Read the model definition and answer for the solid it produces. Units are mm, in the model's axes. A direction names the side the tool comes from. Round coordinates to 2 decimals unless told otherwise and drop trailing zeros. Loops run counter-clockwise (first coordinate to the right, second up) from the corner with the lowest first, then second, coordinate; pieces in that order, holes last. Notation, with made-up numbers: M 54.5,-10 L 63.5,-10 A32 cw 63.5,25 Z; hole C 73.25,41.25 d11. An arc over 180 degrees is marked long. Write each question's results on one line, items separated by ' | '.
Autodesk Inventor part; units mm, degrees
ref_plane "YZ Plane" through (0, 0, 0) normal (1, 0, 0) x (0, 1, 0)
ref_plane "XZ Plane" through (0, 0, 0) normal (0, 1, 0) x (-1, 0, 0)
ref_plane "XY Plane" through (0, 0, 0) normal (0, 0, 1) x (1, 0, 0)
sketch "Sketch2" plane through (0, 0, 0) normal (0, 0, 1) x (1, 0, 0)
  line L0 (-54, 10) -> (54, 10)
  line L1 (55, 9) -> (55, -9)
  line L2 (54, -10) -> (-54, -10)
  line L3 (-55, -9) -> (-55, 9)
  line L4 (-55, 10) -> (55, -10) construction
  line L5 (55, 10) -> (-55, -10) construction
  line L6 (53, 8) -> (-53, 8)
  line L7 (-53, 8) -> (-53, -8)
  line L8 (-53, -8) -> (53, -8)
  line L9 (53, -8) -> (53, 8)
  line L10 (56, 11) -> (-56, 11)
  line L11 (-56, 11) -> (-56, -11)
  line L12 (-56, -11) -> (56, -11)
  line L13 (56, -11) -> (56, 11)
  arc A0 (55, 9) -> (54, 10) centre (54, 9) ccw
  arc A1 (54, -10) -> (55, -9) centre (54, -9) ccw
  arc A2 (-55, -9) -> (-54, -10) centre (-54, -9) ccw
  arc A3 (-54, 10) -> (-55, 9) centre (-54, 9) ccw
  point P0 (0, 0)
  dimension "d0" = 110
  dimension "d1" = 20
  dimension "d2" = 2
  dimension "d3" = 1
  dimension "d10" = 1
extrude "Extrusion2" [suppressed]
sketch "Sketch3" plane through (-56, -11, 0) normal (-1, 0, 0) x (0, 0, 1)
  line L0 (7, 17) -> (9, 17)
  line L1 (9, 17) -> (9, 5)
  line L2 (9, 5) -> (7, 5)
  line L3 (7, 5) -> (7, 17)
  line L4 (0, 22) -> (0, 0)
  line L5 (0, 22) -> (12, 22)
  circle A0 centre (4, 11) radius 2
  line L6 (12, 22) -> (12, 0)
  line L7 (0, 11) -> (2, 11) construction
  dimension "d20" = 4
  dimension "d12" = 2
  dimension "d13" = 12
  dimension "d15" = 5
  dimension "d21" = 3
  dimension "d24" = 4
  dimension "d25" = 2
  dimension "d26" = 3
extrude "Extrusion4" [suppressed]
sketch "Sketch4" plane through (-54, 10, 12) normal (0, -1, 0) x (1, 0, 0)
  line L0 (3.4899, -1) -> (43.4899, -1)
  line L1 (43.4899, -1) -> (43.4899, 0)
  line L2 (43.4899, 0) -> (3.4899, 0)
  line L3 (3.4899, 0) -> (3.4899, -1)
  line L4 (0, 0) -> (108, 0)
  point P0 (54, -12)
  dimension "d27" = 1
  dimension "d28" = 40
extrude "Extrusion6" [suppressed]
ref_plane "Work Plane1" through (-56, -11, 12) normal (0, -1, 0) x (1, 0, 0)
sketch "Sketch5" plane through (-56, -11, 12) normal (0, -1, 0) x (1, 0, 0)
  line L0 (111, -12) -> (111, 0) construction
  line L1 (111, -6) -> (1, -6) construction
  line L2 (1, -12) -> (1, 0) construction
  line L3 (38.5, -3.5) -> (38.5, -8.5)
  line L4 (38.5, -8.5) -> (43.5, -8.5)
  line L5 (43.5, -8.5) -> (43.5, -3.5)
  line L6 (43.5, -3.5) -> (38.5, -3.5)
  line L7 (38.5, -3.5) -> (43.5, -8.5) construction
  line L8 (38.5, -8.5) -> (43.5, -3.5) construction
  line L9 (26.5, -9.5) -> (26.5, -2.5)
  line L10 (26.5, -2.5) -> (33.5, -2.5)
  line L11 (33.5, -2.5) -> (33.5, -9.5)
  line L12 (33.5, -9.5) -> (26.5, -9.5)
  line L13 (26.5, -9.5) -> (33.5, -2.5) construction
  line L14 (26.5, -2.5) -> (33.5, -9.5) construction
  line L15 (60.4912, -8.5) -> (65.4912, -8.5)
  line L16 (65.4912, -8.5) -> (65.4912, -3.5)
  line L17 (65.4912, -3.5) -> (60.4912, -3.5)
  line L18 (60.4912, -3.5) -> (65.4912, -8.5) construction
  line L19 (60.4912, -3.5) -> (60.4912, -8.5)
  line L20 (60.4912, -8.5) -> (65.4912, -3.5) construction
  line L21 (55.4912, -9.5) -> (48.4912, -9.5)
  line L22 (48.4912, -9.5) -> (48.4912, -2.5)
  line L23 (55.4912, -2.5) -> (55.4912, -9.5)
  line L24 (48.4912, -9.5) -> (55.4912, -2.5) construction
  line L25 (48.4912, -2.5) -> (55.4912, -9.5) construction
  line L26 (48.4912, -2.5) -> (55.4912, -2.5)
  line L27 (77.5, -9.5) -> (70.5, -9.5)
  line L28 (77.5, -2.5) -> (77.5, -9.5)
  line L29 (70.5, -2.5) -> (77.5, -2.5)
  line L30 (70.5, -2.5) -> (77.5, -9.5) construction
  line L31 (70.5, -9.5) -> (70.5, -2.5)
  line L32 (70.5, -9.5) -> (77.5, -2.5) construction
  line L33 (82.5, -3.5) -> (82.5, -8.5)
  line L34 (87.5, -3.5) -> (82.5, -3.5)
  line L35 (82.5, -3.5) -> (87.5, -8.5) construction
  line L36 (82.5, -8.5) -> (87.5, -3.5) construction
  line L37 (87.5, -8.5) -> (87.5, -3.5)
  line L38 (82.5, -8.5) -> (87.5, -8.5)
  line L39 (99.5, -9.5) -> (92.5, -9.5)
  line L40 (99.5, -2.5) -> (99.5, -9.5)
  line L41 (92.5, -2.5) -> (99.5, -2.5)
  line L42 (92.5, -2.5) -> (99.5, -9.5) construction
  line L43 (92.5, -9.5) -> (92.5, -2.5)
  line L44 (92.5, -9.5) -> (99.5, -2.5) construction
  line L45 (106, -6) -> (30, -6) construction
  line L46 (110, 0) -> (111, 0)
  line L47 (110, -12) -> (2, -12)
  line L48 (111, 0) -> (21, 0)
  line L49 (21, 0) -> (21, -12)
  line L50 (21, -12) -> (111, -12)
  line L51 (111, -12) -> (111, 0)
  line L52 (112, -14) -> (112, 0)
  line L53 (111, 0) -> (112, 0)
  line L54 (112, 0) -> (112, -14)
  line L55 (112, -14) -> (21, -14)
  line L56 (0, -14) -> (112, -14)
  line L57 (21, -14) -> (21, -12)
  point P0 (41, -6)
  point P1 (62.9912, -6)
  point P2 (51.9912, -6)
  point P3 (74, -6)
  point P4 (85, -6)
  point P5 (96, -6)
  dimension "d47" = 5
  dimension "d48" = 5
  dimension "d49" = 7
  dimension "d50" = 7
  dimension "d51" = 5
  dimension "d52" = 5
  dimension "d53" = 7
  dimension "d54" = 7
  dimension "d55" = 5
  dimension "d56" = 5
  dimension "d57" = 7
  dimension "d58" = 7
  dimension "d59" = 7
  dimension "d60" = 7
  dimension "d61" = 5
  dimension "d62" = 90
  dimension "d63" = 12
extrude "Extrusion7" add sketch "Sketch5" along normal blind 1
extrude "Extrusion8" add sketch "Sketch5" along normal mid plane 30 contours L53 L52 L55 L57 L47 L50 L51
properties part number "sdm_finger_marker_jig"
1. Find section B-B, the plane z = 10.75. Give the vertices of the cut face in (x, y).
Completed:
outline: M -35,-12 L 55,-12 L 55,-26 L 56,-26 L 56,4 L 55,4 L 55,-11 L -35,-11 Z
2. Find section C-C, the plane x = 49. Give the vertices of the cut face in (y, z), then the cut area to 3 significant figures.
Completed:
outline: M -26,-2 L 4,-2 L 4,0 L -11,0 L -11,12 L -12,12 L -12,0 L -26,0 Z | area: 72.0 mm2
3. Given P1, Ø6, axis at x = -14, z = 6, coming from the +Y side; P2, Ø5, axis at y = -18, z = 5, coming from the -X side; P3, Ø5, axis at y = -20.5, z = 2, coming from the -X side; P4, Ø2, axis at x = -12, z = 10.5, coming from the -Y side, each flat-ended and moving along its own axis, determine where each tip first touches the part or whether it passes through.
Completed:
P1: stops at y = -11 | P2: stops at x = 55 | P3: stops at x = -35 | P4: stops at y = -12
4. Which of the six approach directions +Z, -Z, +X, -X, +Y, -Y give full straight-line access (tool end or side, diameter ignored) to faces 1 (the face through (9, -11, 9)), 2 (the face through (56, -11, 5)), 3 (the face through (55, -19, 6))?
Completed:
face 1: +Z, -X, +Y | face 2: +Z, -Z, +X, +Y, -Y | face 3: +Z, -X, -Y
5. Find the intervals of material crossed by L1, parallel to Z at x = 33, y = -21.25; L2, parallel to Y at x = 47.5, z = 1.25; L3, parallel to X at y = -14, z = 8, in increasing order.
Completed:
L1: z = -2 to 0 | L2: y = -12 to -11 | L3: x = 55 to 56
6. Find section D-D, the plane z = 6.25. Count the separate pieces of the cut face and the enclosed holes in it, then the cut area to 3 significant figures.
Completed:
separate pieces: 8 | enclosed holes: 0 | area: 77.0 mm2
7. Find section A-A, the plane x = -5. Give the vertices of the cut face in (y, z).
Completed:
outline: M -26,-2 L 4,-2 L 4,0 L -11,0 L -11,2.5 L -12,2.5 L -12,0 L -26,0 Z; M -12,9.5 L -11,9.5 L -11,12 L -12,12 Z
